Geometry check sheet. Reference: the model listing, model coordinates, mm. A direction names the side the tool comes from. Coordinates: 2 decimals unless noted, no trailing zeros. Order: outer loops, then holes, each group sorted by start corner. A loop starts at its lowest first (then second) coordinate and runs counter-clockwise, first axis right, second up. Notation, with made-up numbers: (15, 8.25) -> (62, 8.25) arc R24 ccw to (62, 46.25) -> close; hole circle Ø5 at (30, 62.5). An arc over 180 degrees is marked (long way). Answer in a Markdown table with one row per item. Add a question column.
```python
from build123d import *

# Parameters (mm, degrees)
SKETCH1_R           = 12.7
BOSS_EXTRUDE1_DEPTH = 89.916
SKETCH2_R           = 8.89
CUT_EXTRUDE1_DEPTH  = 92.69224098
SKETCH3_R           = 10.033
CUT_EXTRUDE2_DEPTH  = 12.7
CUT_EXTRUDE3_START  = -12.192
SKETCH4_R           = 12.7
SKETCH4_R_2         = 10.16
CUT_EXTRUDE3_DEPTH  = 12.192
FILLET1_R           = 1.27
CHAMFER1_SIZE       = 1.27
FILLET2_R           = 0.635
CHAMFER2_SIZE       = 1.27
SKETCH5_R           = 14.986
SKETCH5_R_2         = 12.7
BOSS_EXTRUDE2_DEPTH = 25.4
FILLET3_R           = 2.54
CHAMFER3_SIZE       = 2.54


# Some blends are built 0.0001 mm under size
with BuildPart() as part:
    # Sketch1 → Boss-Extrude1 (new body)
    with BuildSketch(Plane.XY):
        Circle(SKETCH1_R)
    extrude(amount=BOSS_EXTRUDE1_DEPTH)

    # Sketch2 → Cut-Extrude1 (cut, through all)
    with BuildSketch(Plane(origin=(0, 0, 0), x_dir=(-1, 0, 0), z_dir=(0, 0, -1))):
        Circle(SKETCH2_R)
    extrude(amount=-CUT_EXTRUDE1_DEPTH, mode=Mode.SUBTRACT)

    # Sketch3 → Cut-Extrude2 (cut)
    with BuildSketch(Plane(origin=(0, 0, 0), x_dir=(-1, 0, 0), z_dir=(0, 0, -1))):
        Circle(SKETCH3_R)
    extrude(amount=-CUT_EXTRUDE2_DEPTH, mode=Mode.SUBTRACT)

    # Sketch4 → Cut-Extrude3 (cut)
    with BuildSketch(Plane.XY.offset(89.916).offset(CUT_EXTRUDE3_START)):
        Circle(SKETCH4_R)
        Circle(SKETCH4_R_2, mode=Mode.SUBTRACT)
    extrude(amount=CUT_EXTRUDE3_DEPTH, mode=Mode.SUBTRACT)

    # Fillet1
    fillet1_edges = [part.edges().sort_by_distance(p)[0] for p in [
        (-10.16, 0, 77.724),
    ]]
    fillet(fillet1_edges, radius=FILLET1_R)

    # Chamfer1
    chamfer1_edges = [part.edges().sort_by_distance(p)[0] for p in [
        (10.033, 0, 0),
    ]]
    chamfer(chamfer1_edges, length=CHAMFER1_SIZE)

    # Fillet2
    fillet2_edges = [part.edges().sort_by_distance(p)[0] for p in [
        (10.033, 0, 12.7),
    ]]
    fillet(fillet2_edges, radius=FILLET2_R)

    # Chamfer2
    chamfer2_edges = [part.edges().sort_by_distance(p)[0] for p in [
        (-10.16, 0, 89.916),
    ]]
    chamfer(chamfer2_edges, length=CHAMFER2_SIZE - 0.0001)  # a hair under: the kernel refuses the full size

    # Sketch5 → Boss-Extrude2 (add)
    with BuildSketch(Plane(origin=(0, 0, 0), x_dir=(-1, 0, 0), z_dir=(0, 0, -1))):
        Circle(SKETCH5_R)
        Circle(SKETCH5_R_2, mode=Mode.SUBTRACT)
    extrude(amount=-BOSS_EXTRUDE2_DEPTH)

    # Fillet3
    # the kernel refuses this fillet: 2.54 mm, written as the material it adds along each edge
    with BuildSketch(Plane(origin=(0, 0, 25.4), x_dir=(1, 0, 0), z_dir=(0, -1, 0))) as fillet3_piece_1:
        with BuildLine():
            CenterArc((15.24, 2.52726809), FILLET3_R, 180, 84.260829523)
            Line((12.7, 2.52726809), (12.6492, 2.52726809))
            Line((12.6492, 2.52726809), (12.6492, 0))
            Line((12.6492, 0), (12.7, -0.0508))
            ThreePointArc((12.7, -0.0508), (13.843, -0.0508), (14.98092, -0.050545362))
            Line((14.98092, -0.050545362), (14.986, 0))
        make_face()
    revolve(axis=Axis((0, 0, 25.4), (0, 0, 1)))

    # Chamfer3
    chamfer3_edges = [part.edges().sort_by_distance(p)[0] for p in [
        (14.986, 0, 0),
    ]]
    chamfer(chamfer3_edges, length=CHAMFER3_SIZE)


solid = part.part
```
(1) Go/stop test with flat-tipped pins: P1, Ø6, axis at y = -6.5, z = 53, coming from the +X side; P2, Ø1, axis at x = 0, z = 53, coming from the +Y side; P3, Ø6, axis at x = 2, z = 37.5, coming from the -Y side. Record where each tip stops, or that it passes through.
(2) Mould release check, pull along X, two halves, no side actions. Record for faces 4 (the face through (-5.5, -10.1, 0)), 5 (the face through (1.93, -8.68, 50.77)), 6 (the face through (-11.989, 3.775, 0.123)): +X half, -X half, draft (parallel to the pull), parting line (faces both ways), or undercut.
(3) Cross-section at C-C (z = 15.5). Enter the section's corners in (x, y), plus the area to 3 significant figures.
(4) Scan lines: line 1 along Y through (x, z) = (0, 59.5); line 2 along Y through (x, z) = (0, 6); line 3 along Z through (x, y) = (5, 11.25). Record each from-to range of solid material in increasing order.
(5) Cross-section at D-D (z = 81). Enter the section's corners in (x, y), plus the area to 3 significant figures.
(6) Access from +Z, -Z, +X, -X, +Y, -Y to the whole of each face (thin tool, end or side, straight path). Record for faces 1 (the face through (6, -7, 12.7)), 2 (the face through (-2.75, -12.4, 52.48)), 3 (the face through (1.95, 14.86, 13.81)).
Checks:
| question | item | result |
|---|---|---|
| 1 | P1 | x = 12.21 |
| 1 | P2 | y = 12.7 |
| 1 | P3 | y = -12.7 |
| 2 | face 4 | draft |
| 2 | face 5 | undercut |
| 2 | face 6 | parting line |
| 3 | outline | circle Ø29.97 at (0, 0); hole circle Ø17.78 at (0, 0) |
| 3 | area | 457 mm² |
| 4 | line 1 | -12.7 to -8.89, 8.89 to 12.7 |
| 4 | line 2 | -14.99 to -10.03, 10.03 to 14.99 |
| 4 | line 3 | 0 to 77.72 |
| 5 | outline | circle Ø20.32 at (0, 0); hole circle Ø17.78 at (0, 0) |
| 5 | area | 76.0 mm² |
| 6 | face 1 | -Z |
| 6 | face 2 | +Z |
| 6 | face 3 | +Z, -Z |
